from build123d import *

# Parameters (mm, degrees)
F1_DEPTH = 90


with BuildPart() as f1:
    # F0 (on Front) → F1 (new body)
    with BuildSketch(Plane.XZ):
        with BuildLine():
            Line((3.43934, 4.5), (0, 4.5))
            Line((0, 4.5), (-3.43934, 4.5))
            Line((-3.43934, 4.5), (-6, 7.06066))
            Line((-6, 7.06066), (-6, 8.5))
            Line((-6, 8.5), (-3, 8.5))
            Line((-3, 8.5), (-3, 9.5))
            Line((-3, 9.5), (-3.5, 9.5))
            Line((-3.5, 9.5), (-3.5, 10))
            Line((-3.5, 10), (-8.5, 10))
            ThreePointArc((-8.5, 10), (-9.56066, 9.56066), (-10, 8.5))
            Line((-10, 8.5), (-10, 3.5))
            Line((-10, 3.5), (-9.5, 3.5))
            Line((-9.5, 3.5), (-9.5, 3))
            Line((-9.5, 3), (-8.5, 3))
            Line((-8.5, 3), (-8.5, 6))
            Line((-8.5, 6), (-7.06066, 6))
            Line((-7.06066, 6), (-4.5, 3.43934))
            Line((-4.5, 3.43934), (-4.5, 0))
            Line((-4.5, 0), (-4.5, -3.43934))
            Line((-4.5, -3.43934), (-7.06066, -6))
            Line((-7.06066, -6), (-8.5, -6))
            Line((-8.5, -6), (-8.5, -3))
            Line((-8.5, -3), (-9.5, -3))
            Line((-9.5, -3), (-9.5, -3.5))
            Line((-9.5, -3.5), (-10, -3.5))
            Line((-10, -3.5), (-10, -8.5))
            ThreePointArc((-10, -8.5), (-9.56066, -9.56066), (-8.5, -10))
            Line((-8.5, -10), (-3.5, -10))
            Line((-3.5, -10), (-3.5, -9.5))
            Line((-3.5, -9.5), (-3, -9.5))
            Line((-3, -9.5), (-3, -8.5))
            Line((-3, -8.5), (-6, -8.5))
            Line((-6, -8.5), (-6, -7.06066))
            Line((-6, -7.06066), (-3.43934, -4.5))
            Line((-3.43934, -4.5), (0, -4.5))
            Line((0, -4.5), (3.43934, -4.5))
            Line((3.43934, -4.5), (6, -7.06066))
            Line((6, -7.06066), (6, -8.5))
            Line((6, -8.5), (3, -8.5))
            Line((3, -8.5), (3, -9.5))
            Line((3, -9.5), (3.5, -9.5))
            Line((3.5, -9.5), (3.5, -10))
            Line((3.5, -10), (8.5, -10))
            ThreePointArc((8.5, -10), (9.56066, -9.56066), (10, -8.5))
            Line((10, -8.5), (10, -3.5))
            Line((10, -3.5), (9.5, -3.5))
            Line((9.5, -3.5), (9.5, -3))
            Line((9.5, -3), (8.5, -3))
            Line((8.5, -3), (8.5, -6))
            Line((8.5, -6), (7.06066, -6))
            Line((7.06066, -6), (4.5, -3.43934))
            Line((4.5, -3.43934), (4.5, 0))
            Line((4.5, 0), (4.5, 3.43934))
            Line((4.5, 3.43934), (7.06066, 6))
            Line((7.06066, 6), (8.5, 6))
            Line((8.5, 6), (8.5, 3))
            Line((8.5, 3), (9.5, 3))
            Line((9.5, 3), (9.5, 3.5))
            Line((9.5, 3.5), (10, 3.5))
            Line((10, 3.5), (10, 8.5))
            ThreePointArc((10, 8.5), (9.56066, 9.56066), (8.5, 10))
            Line((8.5, 10), (3.5, 10))
            Line((3.5, 10), (3.5, 9.5))
            Line((3.5, 9.5), (3, 9.5))
            Line((3, 9.5), (3, 8.5))
            Line((3, 8.5), (6, 8.5))
            Line((6, 8.5), (6, 7.06066))
            Line((6, 7.06066), (3.43934, 4.5))
        make_face()
        with BuildLine():
            ThreePointArc((-1.340499, 2.401159), (-0.692573, 2.661361), (0, 2.75))
            ThreePointArc((0, 2.75), (0.692573, 2.661361), (1.340499, 2.401159))
            Line((1.340499, 2.401159), (1.962753, 3.023413))
            Line((1.962753, 3.023413), (3.023413, 1.962753))
            Line((3.023413, 1.962753), (2.401159, 1.340499))
            ThreePointArc((2.401159, 1.340499), (2.661361, 0.692573), (2.75, 0))
            ThreePointArc((2.75, 0), (2.661361, -0.692573), (2.401159, -1.340499))
            Line((2.401159, -1.340499), (3.023413, -1.962753))
            Line((3.023413, -1.962753), (1.962753, -3.023413))
            Line((1.962753, -3.023413), (1.340499, -2.401159))
            ThreePointArc((1.340499, -2.401159), (0.692573, -2.661361), (0, -2.75))
            ThreePointArc((0, -2.75), (-0.692573, -2.661361), (-1.340499, -2.401159))
            Line((-1.340499, -2.401159), (-1.962753, -3.023413))
            Line((-1.962753, -3.023413), (-3.023413, -1.962753))
            Line((-3.023413, -1.962753), (-2.401159, -1.340499))
            ThreePointArc((-2.401159, -1.340499), (-2.661361, -0.692573), (-2.75, 0))
            ThreePointArc((-2.75, 0), (-2.661361, 0.692573), (-2.401159, 1.340499))
            Line((-2.401159, 1.340499), (-3.023413, 1.962753))
            Line((-3.023413, 1.962753), (-1.962753, 3.023413))
            Line((-1.962753, 3.023413), (-1.340499, 2.401159))
        make_face(mode=Mode.SUBTRACT)
    extrude(amount=F1_DEPTH)


solid = f1.part
The listing builds one solid part. Answer for the finished solid, in the listing's coordinates (mm). A direction names the side the tool comes from. Give positions to 0.01 mm unless a question says otherwise; leave off trailing zeros. Answer as a JSON object with one key per item and string values.
1. Find the intervals of material crossed by L1, parallel to X at y = -80.5, z = -8.25; L2, parallel to X at y = -16, z = 5.5, in increasing order. Write a range as [from, to].
Determined:
{"L1": "[-10, -6], [6, 10]", "L2": "[-10, -8.5], [-6.56, -4.44], [4.44, 6.56], [8.5, 10]"}
2. For a pull along Z with two mould halves and no side action, classify faces 1 (the flat face through (-8.5, -44, -5)), 2 (the cylindrical face through (-9.57, -44.37, -9.55)), 3 (the flat face through (0, 0, -4)) as pulls with the +Z half, pulls with the -Z half, needs draft (parallel to the pull), parting line crosses it, or undercut.
Determined:
{"face 1": "undercut", "face 2": "pulls with the -Z half", "face 3": "needs draft"}
3. For faces 4 (the flat face through (-6, -44, -8)), 5 (the cylindrical face through (9.57, -44.37, 9.55)), determine the directions among +Z, -Z, +X, -X, +Y, -Y from which every point of the face is accessible in a straight line to the end or side of a thin tool.
Determined:
{"face 4": "+Y, -Y", "face 5": "+Z, +X, +Y, -Y"}
4. Flat-ended cylindrical pins translate along their axes: pin 1 Ø2 at (y, z) = (-42.5, 0) entering from +X; pin 2 Ø0.5 at (y, z) = (-53, -9) entering from -X; pin 3 Ø0.8 at (x, y) = (-9, -48.5) entering from -Z. Find the tip coordinate at first contact, or state that the pin passes through.
Determined:
{"pin 1": "x = 4.5", "pin 2": "x = -9.98", "pin 3": "z = -10"}
